from build123d import *

# Parameters (mm, degrees)
SKETCH1_W      = 210
SKETCH1_H      = 297
EXTRUDE1_DEPTH = 0.2
EXTRUDE2_START = 0.2
EXTRUDE2_DEPTH = 0.1


# Read off the part's stored shape, not the designer's step: Extrude2
with BuildPart() as part:
    # Sketch1 → Extrude1 (new body)
    with BuildSketch(Plane(origin=(0, 0, 0), x_dir=(1, 0, 0), z_dir=(0, 1, 0))):
        with Locations((105, 148.5)):
            Rectangle(SKETCH1_W, SKETCH1_H)
    extrude(amount=EXTRUDE1_DEPTH)

    # Extrude2 outline → Extrude2 (add)
    # profile 1 of 2: a face of its own
    with BuildSketch(Plane(origin=(0, 0, 0), x_dir=(1, 0, 0), z_dir=(0, 1, 0)).offset(EXTRUDE2_START)):
        Polygon((135.38747678, 94.971472029), (152.034111396, 94.971472029), (192.438758831, 194.971472029), (173.288117806, 194.971472029), (165.515681908, 174.458651516), (121.94597037, 174.458651516), (114.173534472, 194.971472029), (95.002861396, 194.971472029), align=None)
        Polygon((158.704784472, 156.509933567), (143.720810113, 121.794388695), (128.736835755, 156.509933567), align=None, mode=Mode.SUBTRACT)
    # profile 2 of 2: a face of its own
    with BuildSketch(Plane(origin=(0, 0, 0), x_dir=(1, 0, 0), z_dir=(0, 1, 0)).offset(EXTRUDE2_START)):
        Polygon((46.925938319, 174.458651516), (46.925938319, 194.971472029), (28.97722037, 194.971472029), (28.97722037, 174.458651516), (20.002861396, 174.458651516), (20.002861396, 157.791984849), (28.97722037, 157.791984849), (28.97722037, 92.407369465), (47.687156267, 92.407369465), (89.233630626, 156.289581003), (89.233630626, 174.458651516), align=None)
        Polygon((69.061354985, 157.791984849), (46.925938319, 123.757529721), (46.925938319, 157.791984849), align=None, mode=Mode.SUBTRACT)
    extrude(amount=EXTRUDE2_DEPTH)


solid = part.part
Design review of the part built by this model. Coordinates are the model's own, in mm. Round coordinates to 2 decimals unless told otherwise and drop trailing zeros. Loops run counter-clockwise (first coordinate to the right, second up) from the corner with the lowest first, then second, coordinate; pieces in that order, holes last. Notation, with made-up numbers: M 68,61 L 81,61 A28 ccw 81,88 Z; hole C 7,30.5 d11. An arc over 180 degrees is marked long. Answer as a JSON object with one key per item and string values.
Item 1: Clearance check with a flat-ended pin moving along its axis: P1, Ø10, axis at x = 57.5, z = -40, coming from the +Y side. State where the tip first meets the part, or that it passes through.
Answer sheet:
{"P1": "stops at y = 0.2"}
Item 2: Wall thickness on L1, parallel to Y at x = 143.5, z = -215; L2, parallel to X at y = 0.25, z = -154; L3, parallel to Z at x = 123, y = 0.25: over which ranges is each line inside the solid? List them lowest first. Write a range as from..to.
Answer sheet:
{"L1": "y = 0..0.2", "L2": "x = 28.98..46.93, 66.6..87.74, 111.55..129.82, 157.62..175.88", "L3": "z = -174.46..-125.65"}
Item 3: We need section C-C on z = -171.5. Give the boundary of the cut face in (x, y).
Answer sheet:
{"outline": "M 0,0 L 210,0 L 210,0.2 L 182.96,0.2 L 182.96,0.3 L 104.48,0.3 L 104.48,0.2 L 89.23,0.2 L 89.23,0.3 L 20,0.3 L 20,0.2 L 0,0.2 Z"}
Item 4: We need section A-A on y = 0.25. Give the boundary of the cut face in (x, z).
Answer sheet:
{"outline": "M 20,-174.46 L 28.98,-174.46 L 28.98,-194.97 L 46.93,-194.97 L 46.93,-174.46 L 89.23,-174.46 L 89.23,-156.29 L 47.69,-92.41 L 28.98,-92.41 L 28.98,-157.79 L 20,-157.79 Z; M 95,-194.97 L 114.17,-194.97 L 121.95,-174.46 L 165.52,-174.46 L 173.29,-194.97 L 192.44,-194.97 L 152.03,-94.97 L 135.39,-94.97 Z; hole M 46.93,-157.79 L 69.06,-157.79 L 46.93,-123.76 Z; hole M 128.74,-156.51 L 158.7,-156.51 L 143.72,-121.79 Z"}
Item 5: We need section B-B on x = 24. Give the boundary of the cut face in (y, z).
Answer sheet:
{"outline": "M 0,-297 L 0.2,-297 L 0.2,-174.46 L 0.3,-174.46 L 0.3,-157.79 L 0.2,-157.79 L 0.2,0 L 0,0 Z"}
Item 6: We need section D-D on x = 85. Give the boundary of the cut face in (y, z).
Answer sheet:
{"outline": "M 0,-297 L 0.2,-297 L 0.2,-174.46 L 0.3,-174.46 L 0.3,-149.78 L 0.2,-149.78 L 0.2,0 L 0,0 Z"}
